For this review, take the finished solid that the model builds, in its own axes (mm). A direction names the side the tool comes from. Round coordinates to 2 decimals unless told otherwise and drop trailing zeros. Write each loop counter-clockwise with the first axis right and the second up, starting at its lowest first coordinate (ties: lowest second). Pieces come first, ordered by that corner, then holes. Notation, with made-up numbers: (73, 9) -> (108, 9) arc R38 ccw to (108, 48) -> close; hole circle Ø3 at (-34.5, 75.25). An arc over 180 degrees is marked (long way). Write item = value, one per line. Start each with the question number.
```python
from build123d import *
from build123d import SkipClean  # not in build123d's __all__

# Parameters (mm, degrees)
F0_R      = 4.16
F1_DEPTH  = 15
F3_DEPTH  = 100
F4_W      = 23.4
F4_H      = 8
F5_DEPTH  = 25
F7_COUNT  = 3
F9_START  = 22
F8_R      = 16.7795
F8_R_2    = 13.7795
F9_DEPTH  = 38
F10_R     = 13.7795
F11_DEPTH = 40
F12_R     = 14.33068
F12_R_2   = 13.7795
F13_DEPTH = 40
F15_DEPTH = 100


# Not quite as in the source:
# - a feature names something its author has since deleted; it is built from what else it names


with BuildPart() as f1:
    # F0 (on Top) → F1 (new body)
    with BuildSketch(Plane.XY):
        Polygon((-33.7795, 0), (-15.7795, 0), (-15.7795, 50), (-15.7795, 100), (-33.7795, 100), (-33.7795, 70), (-23.7483102828, 61), (-23.7483102828, 50), (-23.7483102828, 39), (-33.7795, 30), align=None)
        with Locations((-24.7795, 15)):
            Circle(F0_R, mode=Mode.SUBTRACT)
        with Locations((-24.7795, 85)):
            Circle(F0_R, mode=Mode.SUBTRACT)
    extrude(amount=F1_DEPTH)

    # F2 (on face) → F3 (join)
    with BuildSketch(Plane.XZ):
        with BuildLine():
            ThreePointArc((-7.7342375, -7.9925473083), (-15.468475, 5.4035449996), (-7.7342375, 18.7996373074))
            Line((-7.7342375, 18.7996373074), (-9.2342375, 21.3977135187))
            ThreePointArc((-9.2342375, 21.3977135187), (-12.9094713485, 18.6107444881), (-15.7795, 15))
            Line((-15.7795, 15), (-15.7795, 0))
            Line((-15.7795, 0), (-17.6603021, 0))
            ThreePointArc((-17.6603021, 0), (-14.4523144066, -6.0949408624), (-9.2342375, -10.5906235196))
            Line((-9.2342375, -10.5906235196), (-7.7342375, -7.9925473083))
        make_face()
    extrude(amount=-F3_DEPTH)

    # F4 (on face) → F5 (cut)
    with BuildSketch(Plane(origin=(-33.7795, 0, 0), x_dir=(0, -1, 0), z_dir=(-1, 0, 0))):
        with Locations((-84.9, 7.5)):
            Rectangle(F4_W, F4_H)
        with Locations((-15.1, 7.5)):
            Rectangle(F4_W, F4_H)
    extrude(amount=-F5_DEPTH, mode=Mode.SUBTRACT)

    # F7: F1 ×3 about axis
    f7_axis = Axis((0, 0, 5.4035449996), (0, -1, 0))


with BuildPart() as f1_1:
    add(f1.part, clean=False)
    with SkipClean():  # cleaning this boolean's faces spoils the solid; the shape is the same uncleaned
        for i in range(1, F7_COUNT):
            add(f1.part.rotate(f7_axis, i * 360 / F7_COUNT), clean=False)

    # F8 (on Top) → F9 (join)
    with BuildSketch(Plane.XY.offset(F9_START)):
        with Locations((0, 50)):
            Circle(F8_R)
        with Locations((0, 50)):
            Circle(F8_R_2, mode=Mode.SUBTRACT)
    with SkipClean():  # cleaning this boolean's faces spoils the solid; the shape is the same uncleaned
        extrude(amount=F9_DEPTH)

    # F10 (on face) → F11 (cut)
    with BuildSketch(Plane.XY.offset(60)):
        with Locations((0, 50)):
            Circle(F10_R)
    with SkipClean():  # cleaning this boolean's faces spoils the solid; the shape is the same uncleaned
        extrude(amount=-F11_DEPTH, mode=Mode.SUBTRACT)

    # F12 (on face) → F13 (cut)
    with BuildSketch(Plane.XY.offset(60)):
        with Locations((0, 50)):
            Circle(F12_R)
        with Locations((0, 50)):
            Circle(F12_R_2, mode=Mode.SUBTRACT)
    with SkipClean():  # cleaning this boolean's faces spoils the solid; the shape is the same uncleaned
        extrude(amount=-F13_DEPTH, mode=Mode.SUBTRACT)

    # F14 (on Front) → F15 (cut)
    with BuildSketch(Plane.XZ):
        Polygon((-4.9232800736, -4.035219008), (-6.6853797605, -3.0374381485), (-13.2133684748, -11.2353765363), (-11.6488082544, -12.4812301861), align=None)
    extrude(amount=-F15_DEPTH, mode=Mode.SUBTRACT)


solid = f1_1.part
```
1. Wall thickness on L1, parallel to Z at x = -26, y = 26; L2, parallel to X at y = 15, z = 2.25; L3, parallel to Z at x = 16.5, y = 77: over which ranges is each line inside the solid? List them lowest first. Write a range as from..to.
2. Clearance check with flat-ended pins moving along their axes: pin 1 Ø5 at (x, y) = (-9, 53.5) entering from +Z; pin 2 Ø2 at (x, z) = (-9, -11) entering from +Y; pin 3 Ø3 at (x, y) = (-16, 76) entering from -Z; pin 4 Ø2 at (x, y) = (12, 61) entering from -Z. State where each tip first meets the part, or that it passes through.
3. Consider section B-B, the plane z = 40.5. Give the boundary of the cut face in (x, y), then the cut area to 3 significant figures.
4. Draft analysis for pull direction Y (two halves, no side actions). For faces 5 (the cylindrical face through (-25.68, 10.94, 13.23)), 6 (the flat face through (15.3, 0, 9.2)), 7 (the flat face through (-23, 51, 15)), 8 (the cylindrical face through (8.24, 81.31, 27.04)), state which applies: +Y half, -Y half, draft (parallel to the pull), parting line (faces both ways), or undercut.
5. Machinability: for faces 1 (the flat face through (14, 26.8, 25)), 2 (the flat face through (-28.694, 34.563, 7.395)), 3 (the flat face through (-33.78, 15, 2)), 4 (the flat face through (-24, 73.2, 7)), which of the approach directions +Z, -Z, +X, -X, +Y, -Y give a long, thin tool a straight path to every point of the face, cutting with its end or side? Answer none if there is none.
6. Consider section C-C, the plane y = 31.5. Give the boundary of the cut face in (x, z).
7. Consider section A-A, the plane y = 50. Give the boundary of the cut face in (x, z), then the cut area to 3 significant figures.
8. Consider section D-D, the plane y = 85. Give the number of separate pieces and of enclosed holes in the cut face, then the cut area to 3 significant figures.
Outcome:
q1.L1 = 0..3.5, 11.5..15
q1.L2 = -33.78..-28.94, -20.62..-15.14, 15.14..18.2
q1.L3 = -19.37..-12.37, -2.89..13.7, 14.79..21.79
q2.pin_1 = 20
q2.pin_2 = 100
q2.pin_3 = -6.03
q2.pin_4 = -16.5
q3.outline = circle Ø33.56 at (0, 50); hole circle Ø28.66 at (0, 50)
q3.area = 239 mm2
q4.face_5 = undercut
q4.face_6 = -Y half
q4.face_7 = draft
q4.face_8 = undercut
q5.face_1 = none
q5.face_2 = +Z, -Z, -X
q5.face_3 = +Z, -Z, -X, +Y, -Y
q5.face_4 = -X
q6.outline = (-32.11, 0) -> (-17.66, 0) arc R18.47 ccw to (-11.48, -9.06) -> (-9.61, -6.71) arc R15.47 cw (long way) to (-7.97, -7.86) -> (-9.85, -10.22) arc R18.47 ccw to (-0.42, -13.06) -> (7.74, -27.2) -> (20.73, -19.7) -> (13.51, -7.19) arc R18.47 ccw to (16.2, 14.27) -> (24.36, 28.41) -> (11.37, 35.91) -> (4.15, 23.4) arc R18.47 ccw to (-15.78, 15) -> (-32.11, 15) -> close
q7.outline = (-23.75, 0) -> (-17.66, 0) arc R18.47 ccw to (-11.48, -9.06) -> (-9.61, -6.71) arc R15.47 cw to (-5.12, 20) -> (-11.31, 20) arc R18.47 ccw to (-15.78, 15) -> (-23.75, 15) -> close; (-16.78, 22) -> (-14.33, 22) -> (-14.33, 60) -> (-16.78, 60) -> close; (-9.85, -10.22) arc R18.47 ccw to (-0.42, -13.06) -> (3.56, -19.96) -> (16.55, -12.46) -> (13.51, -7.19) arc R18.47 ccw to (16.2, 14.27) -> (20.18, 21.17) -> (16.78, 23.14) -> (16.78, 60) -> (14.33, 60) -> (14.33, 20) -> (5.12, 20) arc R15.47 cw (long way) to (-7.97, -7.86) -> close
q7.area = 657 mm2
q8.separate_pieces = 10
q8.enclosed_holes = 0
q8.area = 410 mm2
